Could you check a few things on this model? Use its own coordinates, in mm. A direction names the side the tool comes from. Round coordinates to 2 decimals unless told otherwise and drop trailing zeros. Loops run counter-clockwise (first coordinate to the right, second up) from the corner with the lowest first, then second, coordinate; pieces in that order, holes last. Notation, with made-up numbers: (46, -15.5) -> (79, -15.5) arc R33 cw to (79, 18.5) -> close; hole circle Ø2 at (-40, 27.25). An arc over 180 degrees is marked (long way). Write each question's results on one line, items separated by ' | '. Start each with the question number.
1) Imagine slicing it at C-C, the plane y = 40.5. List the corners of the cut face in (x, z) for me, plus the area to 3 significant figures.
2) Imagine slicing it at A-A, the plane x = 19. List the corners of the cut face in (y, z) for me, plus the area to 3 significant figures.
3) Imagine slicing it at B-B, the plane y = 18. List the corners of the cut face in (x, z) for me, plus the area to 3 significant figures.
4) If I drill on probe 1 along Y at (x, z) = (2.5, 0.6); probe 2 along X at (y, z) = (36.5, 1.1); probe 3 along X at (y, z) = (10, 1), over which ranges is the centre line in solid material (lowest first)?
5) Which directions (+Z, -Z, +X, -X, +Y, -Y) give clear straight access to the entire face, cutting with the end or side of a thin tool? Please do faces 4 (the flat face through (0, 3, 2)), 5 (the flat face through (13, 5.969, 2)), 6 (the flat face through (34.798, 3, 2)), 7 (the flat face through (17.399, 10, 2)), 8 (the flat face through (27.559, 15, 2)).
6) For P1, Ø1.1, axis at y = 34, z = 2, coming from the -X side; P2, Ø0.5, axis at y = 22, z = 1, coming from the -X side; P3, Ø1.5, axis at y = 24.5, z = 1, coming from the +X side, each with a flat end and sliding along its axis, tell me the tip position at first contact or that it passes through.
7) We'd pull the mould along Y, two halves only. Please class faces 1 (the flat face through (25.044, 27.153, 1.878)), 2 (the cylindrical face through (0.724, 0.764, 1.932)), 3 (the flat face through (20, 8.954, 2)): pulls with the +Y half, pulls with the -Y half, needs draft (parallel to the pull), parting line crosses it, or undercut.
from build123d import *

# Parameters (mm, degrees)
F0_W     = 5.08
F0_H     = 15.875
F1_DEPTH = 3.81
F2_R     = 2.53999
F3_R     = 0.8382


# Not quite as in the source:
# - two fillets or chamfers of one size are made in one step
# - a fillet or chamfer is up to 0.001 mm smaller than in the source, because OpenCascade refuses the exact size
# - a feature names something its author has since deleted; it is built from what else it names


with BuildPart() as f1:
    # F0 (on Top) → F1 (new body)
    with BuildSketch(Plane.XY):
        Polygon((22.4666253753, 12.2923628866), (17.399, 11.938), (27.559, 11.938), (27.559, 24.638), (22.479, 29.718), (17.399, 29.718), (17.399, 25.908), (22.4666253753, 22.86306348), (22.4666253753, 21.1823628866), (17.399, 20.828), (17.399, 17.018), (22.4666253753, 13.97306348), align=None)
        Polygon((0, 5.969), (0, 0), (34.798, 0), (34.798, 5.969), (27.559, 5.969), (27.559, 11.938), (17.399, 11.938), (17.399, 8.9535), (22.4666253753, 8.9535), (22.4666253753, 5.969), align=None)
        with Locations((19.939, 37.6555)):
            Rectangle(F0_W, F0_H)
    extrude(amount=F1_DEPTH)

    # F2 (radius 2.54 in the source; OpenCascade refuses exactly that, so slightly less here)
    f2_edges = [f1.edges().sort_by_distance(p)[0] for p in [
        (0, 0, 1.905),
        (34.798, 0, 1.905),
        (17.399, 45.593, 1.905),
        (22.479, 45.593, 1.905),
        (0, 5.969, 1.905),
        (34.798, 5.969, 1.905),
        (27.559, 24.638, 1.905),
        (22.479, 29.718, 1.905),
    ]]
    fillet(f2_edges, radius=F2_R)

    # F3
    f3_edges = [f1.edges().sort_by_distance(p)[0] for p in [
        (22.466625, 21.182363, 1.905),
        (22.466625, 22.863063, 1.905),
        (22.466625, 12.292363, 1.905),
        (22.466625, 13.973063, 1.905),
        (17.399, 11.938, 1.905),
        (17.399, 17.018, 1.905),
        (17.399, 20.828, 1.905),
        (17.399, 25.908, 1.905),
    ]]
    fillet(f3_edges, radius=F3_R)


solid = f1.part
Checked values:
1) outline: (17.4, 0) -> (22.48, 0) -> (22.48, 3.81) -> (17.4, 3.81) -> close | area: 19.4 mm^2
2) outline: (0, 0) -> (5.97, 0) -> (5.97, 3.81) -> (0, 3.81) -> close; (8.95, 0) -> (12.05, 0) -> (12.05, 3.81) -> (8.95, 3.81) -> close; (16.06, 0) -> (20.94, 0) -> (20.94, 3.81) -> (16.06, 3.81) -> close; (24.95, 0) -> (45.41, 0) -> (45.41, 3.81) -> (24.95, 3.81) -> close | area: 131 mm^2
3) outline: (17.4, 0) -> (27.56, 0) -> (27.56, 3.81) -> (17.4, 3.81) -> close | area: 38.7 mm^2
4) probe 1: 0 to 5.97 | probe 2: 17.4 to 22.48 | probe 3: 17.4 to 27.56
5) face 4: +Z, -Z, -X, +Y, -Y | face 5: +Z, -Z, -X | face 6: +Z, -Z, +X, +Y, -Y | face 7: +Z, -Z, -X, +Y | face 8: +Z, -Z, +X, +Y
6) P1: x = 17.4 | P2: x = 22.44 | P3: x = 27.55
7) face 1: pulls with the +Y half | face 2: pulls with the -Y half | face 3: undercut
